Could you check a few things on this model? Use its own coordinates, in mm. A direction names the side the tool comes from. Give positions to 0.01 mm unless a question says otherwise; leave off trailing zeros. Write each loop counter-clockwise with the first axis right and the second up, starting at its lowest first coordinate (ties: lowest second). Pieces come first, ordered by that corner, then holes. Notation, with made-up numbers: (-2.75, 71.25) - (12.25, 71.25) arc R21 cw to (12.25, 95.25) - close; hole circle Ø11 at (78, -34). An arc over 180 degrees is marked (long way). Use one line per item in the form item = value.
```python
from build123d import *

# Parameters (mm, degrees)
SKETCH1_W           = 35
SKETCH1_H           = 40
BOSS_EXTRUDE1_DEPTH = 5
SKETCH2_W           = 31
SKETCH2_H           = 36
CUT_EXTRUDE1_DEPTH  = 1
SKETCH3_W           = 35
SKETCH3_H           = 30
BOSS_EXTRUDE2_DEPTH = 5
FILLET2_R           = 3
FILLET3_R           = 3
FILLET4_R           = 3
SKETCH4_W           = 5.036167186
SKETCH4_H           = 5
BOSS_EXTRUDE3_DEPTH = 5


with BuildPart() as part:
    # Sketch1 → Boss-Extrude1 (new body)
    with BuildSketch(Plane(origin=(0, 0, 0), x_dir=(1, 0, 0), z_dir=(0, 1, 0))):
        with Locations((17.5, 20)):
            Rectangle(SKETCH1_W, SKETCH1_H)
    extrude(amount=BOSS_EXTRUDE1_DEPTH)

    # Sketch2 → Cut-Extrude1 (cut)
    with BuildSketch(Plane(origin=(0, 5, 0), x_dir=(1, 0, 0), z_dir=(0, 1, 0))):
        with Locations((17.5, 20)):
            Rectangle(SKETCH2_W, SKETCH2_H)
    extrude(amount=-CUT_EXTRUDE1_DEPTH, mode=Mode.SUBTRACT)

    # Sketch3 → Boss-Extrude2 (add)
    with BuildSketch(Plane.XY):
        with Locations((17.5, 15)):
            Rectangle(SKETCH3_W, SKETCH3_H)
    extrude(amount=BOSS_EXTRUDE2_DEPTH)

    # Fillet2
    fillet2_edges = [part.edges().sort_by_distance(p)[0] for p in [
        (0, 2.5, -40),
    ]]
    fillet(fillet2_edges, radius=FILLET2_R)

    # Fillet3
    fillet3_edges = [part.edges().sort_by_distance(p)[0] for p in [
        (35, 2.5, -40),
    ]]
    fillet(fillet3_edges, radius=FILLET3_R)

    # Fillet4
    fillet4_edges = [part.edges().sort_by_distance(p)[0] for p in [
        (0, 30, 2.5),
        (35, 30, 2.5),
    ]]
    fillet(fillet4_edges, radius=FILLET4_R)

    # Sketch4 → Boss-Extrude3 (add)
    with BuildSketch(Plane.XY.offset(5)):
        with Locations((17.5, 13.5)):
            Rectangle(SKETCH4_W, SKETCH4_H)
    extrude(amount=BOSS_EXTRUDE3_DEPTH)


solid = part.part
```
1. If we mould it in two halves opening along X, with no side actions, what happens to faces 4 (the face through (34.14, 29.1, 2.54)), 5 (the face through (17, 11, 7)), 6 (the face through (17, 4, -20))? For each: pulls with the +X half, pulls with the -X half, needs draft (parallel to the pull), parting line crosses it, or undercut.
Response values:
face_4 = pulls with the +X half
face_5 = needs draft
face_6 = undercut
2. Which directions (+Z, -Z, +X, -X, +Y, -Y) give clear straight access to the entire face, cutting with the end or side of a thin tool? Please do faces 1 (the face through (17, 16, 7)), 2 (the face through (17, 18, 0)), 3 (the face through (14.982, 13, 7)).
Response values:
face_1 = +Z, +X, -X, +Y
face_2 = -Z, +X, -X, +Y
face_3 = +Z, -X, +Y, -Y
3. Imagine slicing it at C-C, the plane y = 3. List the corners of the cut face in (x, z) for me.
Response values:
outline = (0, -37) arc R3 ccw to (3, -40) - (32, -40) arc R3 ccw to (35, -37) - (35, 5) - (0, 5) - close
4. Imagine slicing it at B-B, the plane z = -5. List the corners of the cut face in (x, y) for me, and give its area (3 significant figures).
Response values:
outline = (0, 0) - (35, 0) - (35, 5) - (33, 5) - (33, 4) - (2, 4) - (2, 5) - (0, 5) - close
area = 144 mm²
5. If I drill on line 1 (Y direction, x = 22, z = -22); line 2 (Z direction, x = 4, y = 25); line 3 (Z direction, x = 19, y = 13.25), over which ranges is the centre line in solid material (lowest first)? Write a range as from..to.
Response values:
line_1 = 0..4
line_2 = 0..5
line_3 = 0..10
6. Imagine slicing it at D-D, the plane y = 21. List the corners of the cut face in (x, z) for me.
Response values:
outline = (0, 0) - (35, 0) - (35, 5) - (0, 5) - close
7. Imagine slicing it at A-A, the plane x = 24. List the corners of the cut face in (y, z) for me, and give its area (3 significant figures).
Response values:
outline = (0, -40) - (5, -40) - (5, -38) - (4, -38) - (4, -2) - (5, -2) - (5, 0) - (30, 0) - (30, 5) - (0, 5) - close
area = 314 mm²
8. For pin 1 (12 mm diameter, centred on x = 28, z = -21.5, fed in from +Y); pin 2 (10 mm diameter, centred on x = 12.5, y = 27, fed in from -Z); pin 3 (6 mm diameter, centred on x = 5.5, y = 25, fed in from +Z), each with a flat end and sliding along its axis, tell me the tip position at first contact or that it passes through.
Response values:
pin_1 = 5
pin_2 = 0
pin_3 = 5
